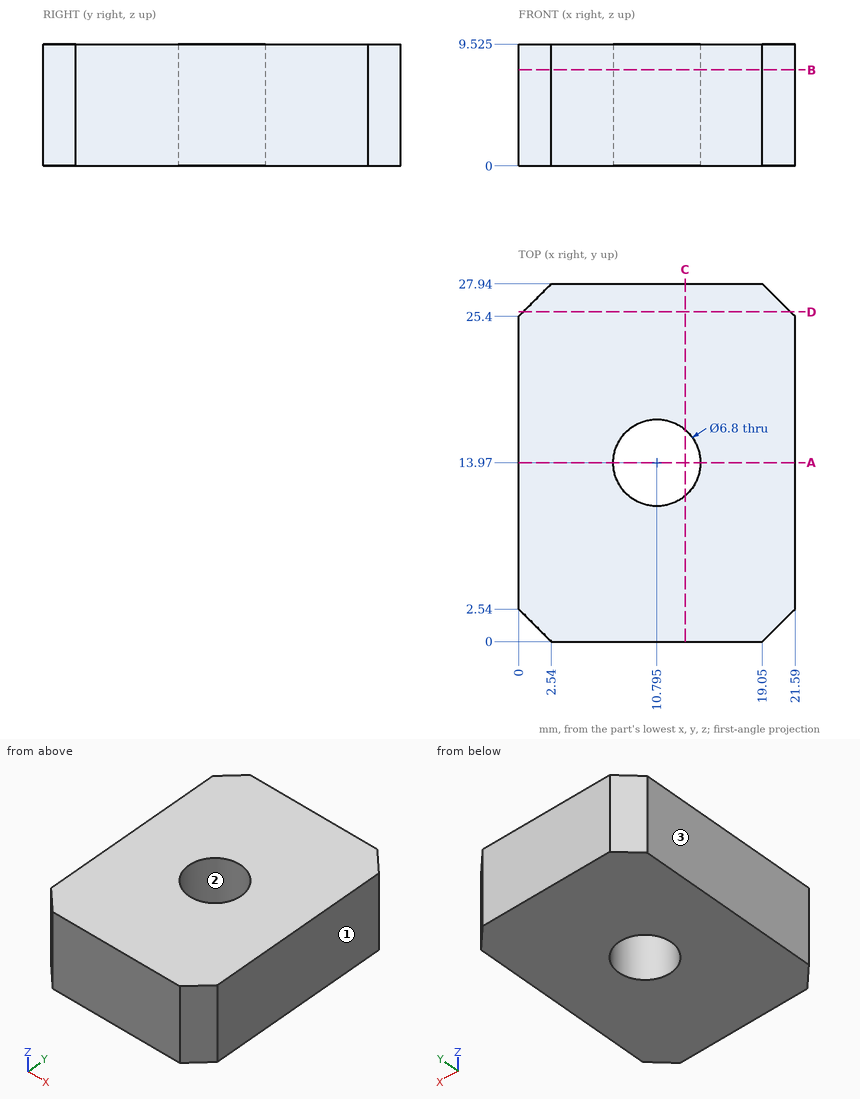
Geometry check sheet. Reference: drawing and pictorial views, mm from the part's lowest x, y, z. Coordinates: 2 decimals unless noted, no trailing zeros. Loops run counter-clockwise (first coordinate to the right, second up) from the corner with the lowest first, then second, coordinate; pieces in that order, holes last.
1) Sectioned sample at D-D (y = 25.75). Record the boundary of the cut face in (x, z) (3 decimals), and give its area (3 significant figures).
2) Sectioned sample at B-B (z = 7.5). Record the boundary of the cut face in (x, y) (3 decimals), and give its area (3 significant figures).
3) Release check for a two-part mould opening along X. For the marked faces 1, 2 and 3 record: released by +X, released by -X, zero draft, split by the parting line, or undercut.
4) Sectioned sample at A-A (y = 13.97). Record the boundary of the cut face in (x, z) (3 decimals), and give its area (3 significant figures).
5) Sectioned sample at C-C (x = 13). Record the boundary of the cut face in (y, z) (3 decimals), and give its area (3 significant figures).
6) Gauge pin test, flat end, axial feed: pin 1 (5.5 mm diameter, centred on x = 10.795, y = 13.97, fed in from +Z). Record the tip position at first contact, or that the pin passes through.
7) Material ranges on probe 1 along X at (y, z) = (12.5, 2.5); probe 2 along X at (y, z) = (11.75, 8); probe 3 along Y at (x, z) = (13.5, 4.25), recorded low to high.
Check sheet entries:
1. outline: (0.35, 0) - (21.24, 0) - (21.24, 9.525) - (0.35, 9.525) - close
1. area: 199 mm2
2. outline: (0, 2.54) - (2.54, 0) - (19.05, 0) - (21.59, 2.54) - (21.59, 25.4) - (19.05, 27.94) - (2.54, 27.94) - (0, 25.4) - close; hole circle Ø6.8 at (10.795, 13.97)
2. area: 554 mm2
3. face 1: released by +X
3. face 2: undercut
3. face 3: released by -X
4. outline: (0, 0) - (7.395, 0) - (7.395, 9.525) - (0, 9.525) - close; (14.195, 0) - (21.59, 0) - (21.59, 9.525) - (14.195, 9.525) - close
4. area: 141 mm2
5. outline: (0, 0) - (11.382, 0) - (11.382, 9.525) - (0, 9.525) - close; (16.558, 0) - (27.94, 0) - (27.94, 9.525) - (16.558, 9.525) - close
5. area: 217 mm2
6. pin 1: passes through
7. probe 1: x = 0 to 7.73, 13.86 to 21.59
7. probe 2: x = 0 to 8.22, 13.37 to 21.59
7. probe 3: y = 0 to 11.91, 16.03 to 27.94
